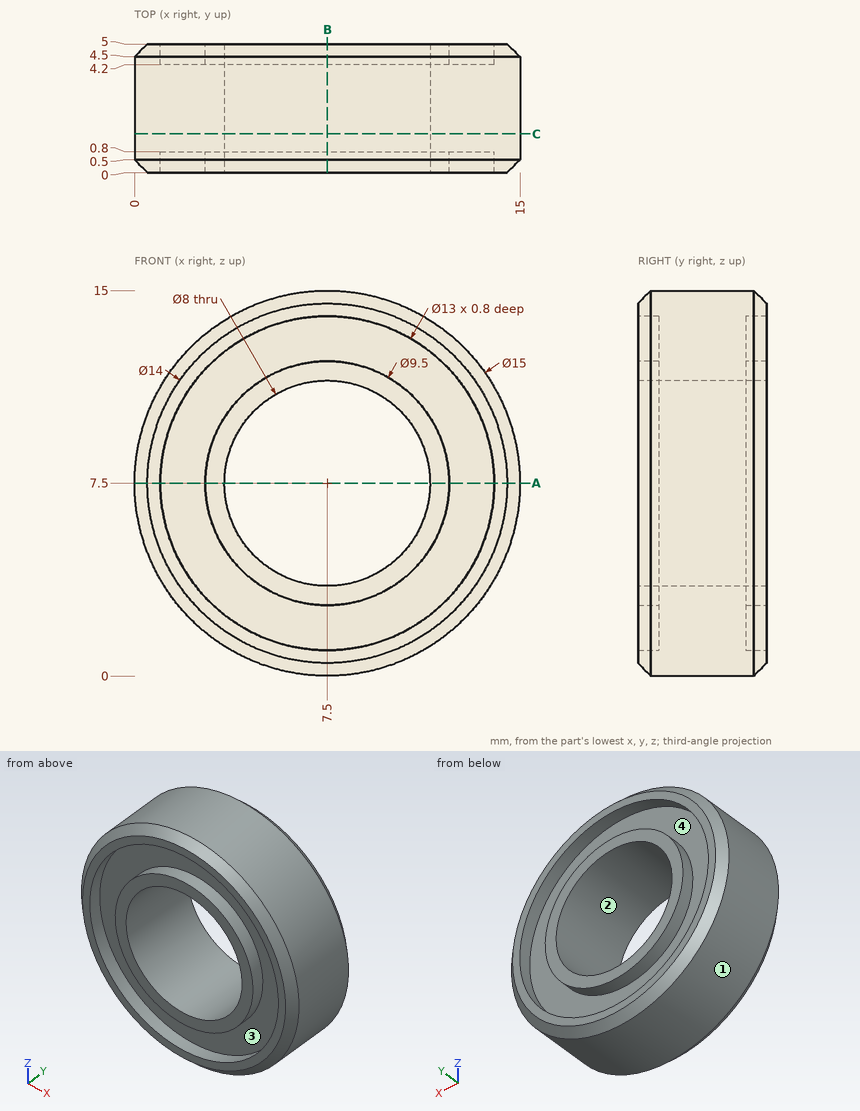
Print and shaded views of the part. All mm, measured from the part's lowest x, y and z. A direction names the side the tool comes from. Round coordinates to 2 decimals unless told otherwise and drop trailing zeros. Write each loop counter-clockwise with the first axis right and the second up, starting at its lowest first coordinate (ties: lowest second). Pieces come first, ordered by that corner, then holes.
(1) Probe line 1 along X through (y, z) = (4.8, 10.25); line 2 along Z through (x, y) = (8.5, 4.3); line 3 along X through (y, z) = (4.45, 11). List the from-to ranges inside material, lowest first.
(2) Slice it at B-B, the plane x = 7.5. Write the cut outline in (y, z), and give its area (3 significant figures).
(3) Slice it at C-C, the plane y = 1.5. Write the cut outline in (x, z), and give its area (3 significant figures).
(4) Slice it at A-A, the plane z = 7.5. Write the cut outline in (x, y).
(5) Drop flat-ended pins along their axis: P1, Ø1, axis at y = 0.5, z = 4.5, coming from the +X side; P2, Ø4, axis at x = 9, z = 7.5, coming from the -Y side. Give the stop position or say it passes through.
(6) Mould opens along X. For the marked faces 1 and 2 say: pulls with the +X half, pulls with the -X half, needs draft (parallel to the pull), parting line crosses it, or undercut.
(7) 3-axis set-ups, long thin cutter, end or side, ignore diameter. For the marked faces 3 and 4: which of +Z, -Z, +X, -X, +Y, -Y reach the whole face in a straight line?
From the geometry:
1. line 1: x = 0.85 to 1.61, 3.63 to 4.6, 10.4 to 11.37, 13.39 to 14.15
1. line 2: z = 0.07 to 1.08, 2.86 to 3.63, 11.37 to 12.14, 13.92 to 14.93
1. line 3: x = 0.87 to 2.02, 4.29 to 5.56, 9.44 to 10.71, 12.98 to 14.13
2. outline: (0, 0.5) - (0.5, 0) - (4.5, 0) - (5, 0.5) - (5, 1) - (4.2, 1) - (4.2, 2.75) - (5, 2.75) - (5, 3.5) - (0, 3.5) - (0, 2.75) - (0.8, 2.75) - (0.8, 1) - (0, 1) - close; (0, 11.5) - (5, 11.5) - (5, 12.25) - (4.2, 12.25) - (4.2, 14) - (5, 14) - (5, 14.5) - (4.5, 15) - (0.5, 15) - (0, 14.5) - (0, 14) - (0.8, 14) - (0.8, 12.25) - (0, 12.25) - close
2. area: 28.9 mm2
3. outline: circle Ø15 at (7.5, 7.5); hole circle Ø8 at (7.5, 7.5)
3. area: 126 mm2
4. outline: (0, 0.5) - (0.5, 0) - (1, 0) - (1, 0.8) - (2.75, 0.8) - (2.75, 0) - (3.5, 0) - (3.5, 5) - (2.75, 5) - (2.75, 4.2) - (1, 4.2) - (1, 5) - (0.5, 5) - (0, 4.5) - close; (11.5, 0) - (12.25, 0) - (12.25, 0.8) - (14, 0.8) - (14, 0) - (14.5, 0) - (15, 0.5) - (15, 4.5) - (14.5, 5) - (14, 5) - (14, 4.2) - (12.25, 4.2) - (12.25, 5) - (11.5, 5) - close
5. P1: stops at x = 14.57
5. P2: passes through
6. face 1: parting line crosses it
6. face 2: undercut
7. face 3: -Y
7. face 4: +Y
